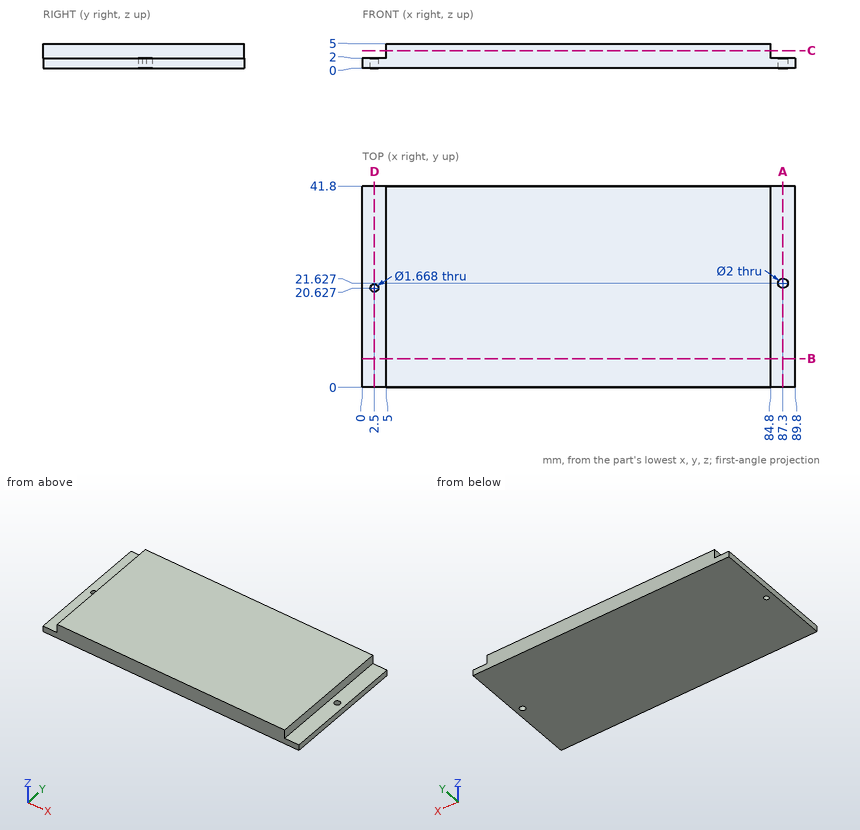
Drawing for the job (mm, zero at the part's lowest x, y, z). Give positions to 0.01 mm unless a question says otherwise; leave off trailing zeros. Loops run counter-clockwise (first coordinate to the right, second up) from the corner with the lowest first, then second, coordinate; pieces in that order, holes last.
Item 1: Slice it at C-C (z = 3.6). Write the cut outline in (x, y).
Check values:
outline: (5, 0) - (84.8, 0) - (84.8, 41.8) - (5, 41.8) - close
Item 2: Drop flat-ended pins along their axis: P1, Ø1.5, axis at x = 2.5, y = 15, coming from the +Z side; P2, Ø2.5, axis at y = 23, z = 4, coming from the -X side; P3, Ø2.5, axis at y = 23, z = 4, coming from the +X side; P4, Ø1, axis at x = 2.5, y = 20.63, coming from the +Z side. Give the stop position or say it passes through.
Check values:
P1: stops at z = 2
P2: stops at x = 5
P3: stops at x = 84.8
P4: passes through
Item 3: Drill centre lines: line 1 along Y through (x, z) = (2.5, 1.1); line 2 along Y through (x, z) = (87.3, 1.5); line 3 along X through (y, z) = (26, 3.3). Where is each one in solid material? Low to high.
Check values:
line 1: y = 0 to 19.79, 21.46 to 41.8
line 2: y = 0 to 20.63, 22.63 to 41.8
line 3: x = 5 to 84.8
Item 4: Slice it at A-A (x = 87.3). Write the cut outline in (y, z), plus the area to 3 significant figures.
Check values:
outline: (0, 0) - (20.63, 0) - (20.63, 2) - (0, 2) - close; (22.63, 0) - (41.8, 0) - (41.8, 2) - (22.63, 2) - close
area: 79.6 mm2
Item 5: Slice it at D-D (x = 2.5). Write the cut outline in (y, z).
Check values:
outline: (0, 0) - (19.79, 0) - (19.79, 2) - (0, 2) - close; (21.46, 0) - (41.8, 0) - (41.8, 2) - (21.46, 2) - close
Item 6: Slice it at B-B (y = 6). Write the cut outline in (x, z).
Check values:
outline: (0, 0) - (89.8, 0) - (89.8, 2) - (84.8, 2) - (84.8, 5) - (5, 5) - (5, 2) - (0, 2) - close
